Design review of the part shown in the three views and the two pictorial views. Dimensions are in mm from the part's minimum x, y and z. Round coordinates to 2 decimals unless told otherwise and drop trailing zeros. Order: outer loops, then holes, each group sorted by start corner. A loop starts at its lowest first (then second) coordinate and runs counter-clockwise, first axis right, second up.
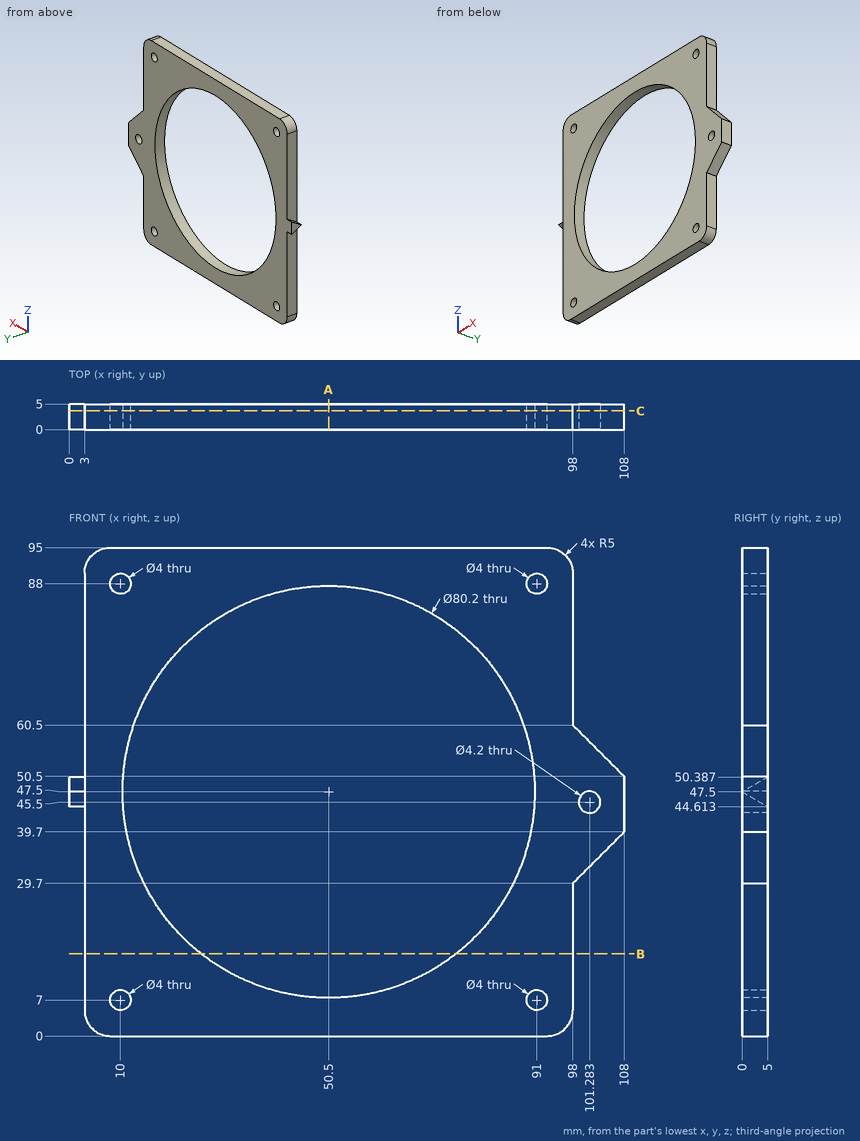
1) To check wall thickness, follow line 1 along X through (y, z) = (4.05, 7); line 2 along Z through (x, y) = (10, 2.35); line 3 along X through (y, z) = (1.9, 45.5). State the ranges of each line that lie inside material, in increasing order.
Results:
line 1: x = 3 to 8, 12 to 89, 93 to 98
line 2: z = 0 to 5, 9 to 86, 90 to 95
line 3: x = 3 to 10.45, 90.55 to 99.18, 103.38 to 108
2) Clearance check with flat-ended pins moving along their axes: P1, Ø1.5, axis at y = 3, z = 20, coming from the +X side; P2, Ø2.5, axis at x = 10, z = 7, coming from the -Y side; P3, Ø2.5, axis at y = 3, z = 31, coming from the -X side. State where each tip first meets the part, or that it passes through.
Results:
P1: stops at x = 98
P2: passes through
P3: stops at x = 3
3) Take a section at B-B on z = 16. Give the boundary of the cut face in (x, y) (1 decimal), plus the area to 3 significant figures.
Results:
outline: (3, 0) - (25.7, 0) - (25.7, 5) - (3, 5) - close; (75.3, 0) - (98, 0) - (98, 5) - (75.3, 5) - close
area: 227 mm2
4) Take a section at C-C on y = 3.65. State how many separate pieces and enclosed holes the cut face has, plus the area to 3 significant figures.
Results:
separate pieces: 1
enclosed holes: 6
area: 4,110 mm2
5) Take a section at A-A on x = 50.5. Give the boundary of the cut face in (y, z).
Results:
outline: (0, 0) - (5, 0) - (5, 7.4) - (0, 7.4) - close; (0, 87.6) - (5, 87.6) - (5, 95) - (0, 95) - close
